Read the model definition and answer for the solid it produces. Units are mm, in the model's axes. Face numbers are marked on the shaded views. Give positions to 0.01 mm unless a question says otherwise; leave off trailing zeros. Loops run counter-clockwise (first coordinate to the right, second up) from the corner with the lowest first, then second, coordinate; pieces in that order, holes last. Notation, with made-up numbers: (-26.5, 18) - (24.5, 18) arc R19 ccw to (24.5, 49) - close; hole circle Ø4 at (69.25, 88). An arc over 180 degrees is marked (long way). Use a Markdown table: item, result. Add a question column.
Item 1: For a pull along Y with two mould halves and no side action, classify the marked faces 1, 2, 3 and 4 as +Y half, -Y half, draft (parallel to the pull), parting line (faces both ways), or undercut.
Item 2: Consider probe 1 along Y at (x, z) = (15, 0.85); probe 2 along Y at (x, z) = (15, 7); probe 3 along X at (y, z) = (7.75, 4). Determine where each line is inside the solid, lowest interval first. Write a range as [from, to].
Item 3: Each of these flat-tipped pins is pushed along its axis until it touches: P1, Ø8, axis at x = 9, y = 9, coming from the +Z side; P2, Ø15, axis at x = 15, y = 15, coming from the +Z side. Where does it stop, or does it pass through?
Item 4: A cutting plane is placed at A-A (x = 15). Determine the outline of the cut face in (y, z), plus the area to 3 significant figures.
Item 5: A cutting plane is placed at B-B (y = 15). Determine the outline of the cut face in (x, z).
Item 6: A cutting plane is placed at D-D (y = 4). Determine the outline of the cut face in (x, z).
Item 7: A cutting plane is placed at C-C (z = 5.5). Determine the outline of the cut face in (x, y), plus the area to 3 significant figures.
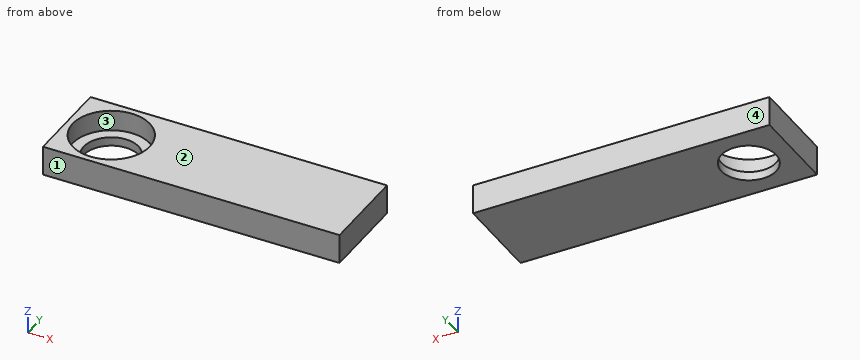
from build123d import *

# Parameters (mm, degrees)
ESBO_O1_W                = 100
ESBO_O1_H                = 30
RESSALTO_EXTRUS_O1_DEPTH = 10
ESBO_O2_R                = 13
CORTE_EXTRUS_O1_DEPTH    = 7
ESBO_O4_R                = 9.25
CORTE_EXTRUS_O3_DEPTH    = 105.637469388
ESBO_O3_W                = 30
ESBO_O3_H                = 30
CORTE_EXTRUS_O2_DEPTH    = 2


with BuildPart() as part:
    # Esboço1 → Ressalto-extrusão1 (new body)
    with BuildSketch(Plane.XY):
        with Locations((50, 15)):
            Rectangle(ESBO_O1_W, ESBO_O1_H)
    extrude(amount=RESSALTO_EXTRUS_O1_DEPTH)

    # Esboço2 → Corte-extrusão1 (cut)
    with BuildSketch(Plane.XY.offset(10)):
        with Locations((15, 15)):
            Circle(ESBO_O2_R)
    extrude(amount=-CORTE_EXTRUS_O1_DEPTH, mode=Mode.SUBTRACT)

    # Esboço4 → Corte-extrusão3 (cut, through all)
    with BuildSketch(Plane.XY.offset(3)):
        with Locations((15, 15)):
            Circle(ESBO_O4_R)
    extrude(amount=-CORTE_EXTRUS_O3_DEPTH, mode=Mode.SUBTRACT)

    # Esboço3 → Corte-extrusão2 (cut)
    with BuildSketch(Plane.XY.offset(10)):
        with Locations((-35, 3.5)):
            Rectangle(ESBO_O3_W, ESBO_O3_H)
    extrude(amount=-CORTE_EXTRUS_O2_DEPTH, mode=Mode.SUBTRACT)


solid = part.part
Geometry says:
| question | item | result |
|---|---|---|
| 1 | face 1 | -Y half |
| 1 | face 2 | draft |
| 1 | face 3 | undercut |
| 1 | face 4 | +Y half |
| 2 | probe 1 | [0, 5.75], [24.25, 30] |
| 2 | probe 2 | [0, 2], [28, 30] |
| 2 | probe 3 | [0, 4.21], [25.79, 100] |
| 3 | P1 | z = 3 |
| 3 | P2 | through |
| 4 | outline | (0, 0) - (5.75, 0) - (5.75, 3) - (2, 3) - (2, 10) - (0, 10) - close; (24.25, 0) - (30, 0) - (30, 10) - (28, 10) - (28, 3) - (24.25, 3) - close |
| 4 | area | 62.5 mm² |
| 5 | outline | (0, 0) - (5.75, 0) - (5.75, 3) - (2, 3) - (2, 10) - (0, 10) - close; (24.25, 0) - (100, 0) - (100, 10) - (28, 10) - (28, 3) - (24.25, 3) - close |
| 6 | outline | (0, 0) - (100, 0) - (100, 10) - (21.93, 10) - (21.93, 3) - (8.07, 3) - (8.07, 10) - (0, 10) - close |
| 7 | outline | (0, 0) - (100, 0) - (100, 30) - (0, 30) - close; hole circle Ø26 at (15, 15) |
| 7 | area | 2,470 mm² |
